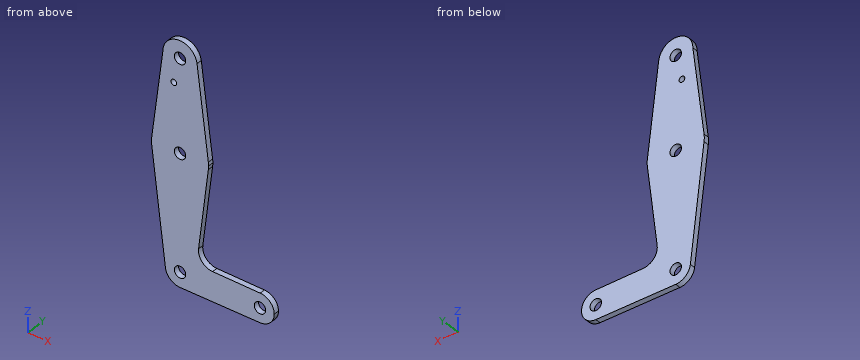
from build123d import *

# Parameters (mm, degrees)
F0_R     = 3.175
F0_R_2   = 1.5875
F1_DEPTH = 3.048


with BuildPart() as f1:
    # F0 (on Front) → F1 (new body)
    with BuildSketch(Plane.XZ):
        with BuildLine():
            ThreePointArc((-9.5248581599, 83.2599219897), (0.0259906378, 73.786938532), (9.525, 83.3119030719))
            ThreePointArc((9.525, 83.3119030719), (9.5063041404, 83.9083983282), (9.4502899547, 84.502551959))
            ThreePointArc((9.4502899547, 84.502551959), (-0.6224326586, 92.8165441795), (-9.5248581599, 83.2599219897))
        make_face()
        with Locations((0, 83.3119030719)):
            Circle(F0_R, mode=Mode.SUBTRACT)
        with BuildLine():
            ThreePointArc((9.4502899547, 84.502551959), (9.5063041404, 83.9083983282), (9.525, 83.3119030719))
            ThreePointArc((9.525, 83.3119030719), (0.0259906378, 73.786938532), (-9.5248581599, 83.2599219897))
            Line((-9.5248581599, 83.2599219897), (-15.7471769435, 34.5234055887))
            ThreePointArc((-15.7471769435, 34.5234055887), (0.0131386883, 48.3879167992), (15.7504832578, 34.4973370481))
            Line((15.7504832578, 34.4973370481), (9.4502899547, 84.502551959))
        make_face()
        with Locations((-3.4761622082, 69.0381222362)):
            Circle(F0_R_2, mode=Mode.SUBTRACT)
        with BuildLine():
            Line((15.7504832578, 30.5285074243), (15.7504832578, 34.4973370481))
            ThreePointArc((15.7504832578, 34.4973370481), (0.0131386883, 48.3879167992), (-15.7471769435, 34.5234055887))
            Line((-15.7471769435, 34.5234055887), (-15.7471769435, 30.5024388837))
            ThreePointArc((-15.7471769435, 30.5024388837), (0.0131386883, 16.6379276732), (15.7504832578, 30.5285074243))
        make_face()
        with Locations((0, 32.5129222362)):
            Circle(F0_R, mode=Mode.SUBTRACT)
        with BuildLine():
            ThreePointArc((15.875, 32.5129222362), (15.8438402339, 33.5070809968), (15.7504832578, 34.4973370481))
            Line((15.7504832578, 34.4973370481), (15.7504832578, 30.5285074243))
            ThreePointArc((15.7504832578, 30.5285074243), (15.8438402339, 31.5187634756), (15.875, 32.5129222362))
        make_face()
        with BuildLine():
            Line((-15.7471769435, 30.5024388837), (-15.7471769435, 34.5234055887))
            ThreePointArc((-15.7471769435, 34.5234055887), (-15.875, 32.5129222362), (-15.7471769435, 30.5024388837))
        make_face()
        with BuildLine():
            Line((10.3100811991, -14.091878104), (15.7504832578, 30.5285074243))
            ThreePointArc((15.7504832578, 30.5285074243), (0.0131386883, 16.6379276732), (-15.7471769435, 30.5024388837))
            Line((-15.7471769435, 30.5024388837), (-8.1291402981, -31.9792369364))
            ThreePointArc((-8.1291402981, -31.9792369364), (-0.4964832457, -22.813821126), (8.1893394424, -30.9880969281))
            ThreePointArc((8.1893394424, -30.9880969281), (5.7907374532, -36.7788343813), (0, -39.1774363705))
            Line((0, -39.1774363705), (44.45, -39.1774363705))
            ThreePointArc((44.45, -39.1774363705), (36.5126271282, -31.1950126056), (44.5398460907, -23.3029448794))
            Line((44.5398460907, -23.3029448794), (18.1118481639, -23.003782117))
            ThreePointArc((18.1118481639, -23.003782117), (12.2199839317, -20.2907985961), (10.3100811991, -14.091878104))
        make_face()
        with BuildLine():
            ThreePointArc((8.1893394424, -30.9880969281), (-0.4964832457, -22.813821126), (-8.1291402981, -31.9792369364))
            ThreePointArc((-8.1291402981, -31.9792369364), (-5.4290191812, -37.1192494489), (0, -39.1774363705))
            ThreePointArc((0, -39.1774363705), (5.7907374532, -36.7788343813), (8.1893394424, -30.9880969281))
        make_face()
        with Locations((0, -30.9880969281)):
            Circle(F0_R, mode=Mode.SUBTRACT)
        with BuildLine():
            ThreePointArc((52.3875, -31.2399363705), (50.0943360812, -25.6591320869), (44.5398460907, -23.3029448794))
            ThreePointArc((44.5398460907, -23.3029448794), (36.5126271282, -31.1950126056), (44.45, -39.1774363705))
            ThreePointArc((44.45, -39.1774363705), (50.0626600757, -36.8525964462), (52.3875, -31.2399363705))
        make_face()
        with Locations((44.45, -31.2399363705)):
            Circle(F0_R, mode=Mode.SUBTRACT)
    extrude(amount=F1_DEPTH)


solid = f1.part
Verification items for the finished model (mm, model axes). Round coordinates to 2 decimals unless told otherwise and drop trailing zeros. Order: outer loops, then holes, each group sorted by start corner. A loop starts at its lowest first (then second) coordinate and runs counter-clockwise, first axis right, second up.
1. Section check A-A on x = 43. Record the cut outline in (y, z).
Final values:
outline: (-3.05, -39.18) - (0, -39.18) - (0, -34.06) - (-3.05, -34.06) - close; (-3.05, -28.42) - (0, -28.42) - (0, -23.29) - (-3.05, -23.29) - close
2. Section check C-C on y = -1.55. State how many separate pieces and enclosed holes the cut face has, then the cut area to 3 significant figures.
Final values:
separate pieces: 1
enclosed holes: 5
area: 3,660 mm2
3. Thickness scan on L1, parallel to X at y = -1.65, z = -33; L2, parallel to Z at x = 2, y = -0.75; L3, parallel to Z at x = 20, y = -2.25. Record the ranges inside material, lowest first.
Final values:
L1: x = -7.94 to -2.46, 2.46 to 41.81, 47.09 to 52.19
L2: z = -39.18 to -33.45, -28.52 to 30.05, 34.98 to 80.85, 85.78 to 92.62
L3: z = -39.18 to -23.03
4. Section check B-B on z = -29.5. Record the cut outline in (x, y).
Final values:
outline: (-8.43, -3.05) - (-2.8, -3.05) - (-2.8, 0) - (-8.43, 0) - close; (2.8, -3.05) - (41.79, -3.05) - (41.79, 0) - (2.8, 0) - close; (47.11, -3.05) - (52.19, -3.05) - (52.19, 0) - (47.11, 0) - close
5. Section check D-D on x = 22. Record the cut outline in (y, z).
Final values:
outline: (-3.05, -39.18) - (0, -39.18) - (0, -23.05) - (-3.05, -23.05) - close
6. Go/stop test with a flat-tipped pin: P1, Ø4, axis at x = 0, z = -30.99, coming from the +Y side. Record where the tip stops, or that it passes through.
Final values:
P1: passes through
